Can you work these out from the model? Positions are in its coordinate system, mm. Face numbers are marked on the shaded views. A direction names the side the tool comes from. Round coordinates to 2 decimals unless told otherwise and drop trailing zeros. Loops run counter-clockwise (first coordinate to the right, second up) from the corner with the lowest first, then second, coordinate; pieces in that order, holes last. Notation, with made-up numbers: (69, 87) -> (87, 87) arc R26 cw to (87, 108) -> close; hole circle Ø9 at (62, -31). An arc over 180 degrees is marked (long way). Write each question's results on one line, items separated by ' | '.
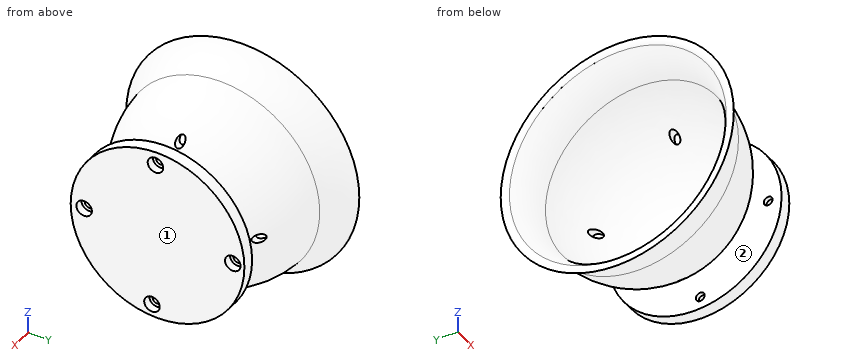
Autodesk Inventor part; units mm, degrees
ref_plane "YZ Plane" through (0, 0, 0) normal (1, 0, 0) x (0, 1, 0)
ref_plane "XZ Plane" through (0, 0, 0) normal (0, 1, 0) x (-1, 0, 0)
ref_plane "XY Plane" through (0, 0, 0) normal (0, 0, 1) x (1, 0, 0)
sketch "Sketch1" plane through (0, 0, 0) normal (0, 1, 0) x (-1, 0, 0)
  arc A0 (-48.26, 0) -> (-2.8901, -48.1734) centre (0, 0) ccw
  line L0 (0, 0) -> (2.3486, 0) construction
  arc A1 (-48.26, -15.8623) -> (-2.7486, -50.7256) centre (0, 0) ccw
  arc A2 (15.4672, -59.6495) -> (-2.7486, -50.7256) centre (-4.1531, -76.6458) ccw
  arc A3 (14.9178, -55.5155) -> (-2.8901, -48.1734) centre (-4.6642, -77.7436) ccw
  arc A4 (15.4672, -59.6495) -> (14.9178, -55.5155) centre (12.8191, -57.8979) ccw
  line L1 (31.2133, 0) -> (-72.6552, 0)
  line L2 (-48.26, 0) -> (-54.61, 0)
  line L3 (-54.61, 0) -> (-54.61, -44.45)
  line L4 (-54.61, -44.45) -> (-48.26, -44.45)
  line L5 (-48.26, -44.45) -> (-48.26, -15.8623)
  point P0 (-50.8, 0)
  dimension "d0" = 48.26
  dimension "d2" = 2.54
  dimension "d3" = 3.175
  dimension "d13" = 6.35
  dimension "d14" = 44.45
  dimension "d15" = 25.9583
  dimension "d16" = 29.6234
  dimension "d17" = 59.6495
  dimension "d18" = 55.5155
  dimension "d19" = 57.8979
  dimension "d20" = 50.6086
  dimension "d21" = 2.54
revolve "Revolution1" add sketch "Sketch1" angle 360 about axis through (-10, 0, 0) along (1, 0, 0)
hole "Hole1" at (54.61, -2.8557, -38.0756) direction (-1, 0, 0) diameter 4.4958 end through all counterbore diameter 7.9502 counterbore depth 4.1656
hole "Hole2" at (54.61, -1.0655, 37.4744) direction (-1, 0, 0) diameter 4.4958 end through all counterbore diameter 7.9502 counterbore depth 4.1656
hole "Hole3" at (54.61, -37.5872, 0.0574) direction (-1, 0, 0) diameter 4.4958 end through all counterbore diameter 7.9502 counterbore depth 4.1656
hole "Hole4" at (54.61, 38.4998, -0.1216) direction (-1, 0, 0) diameter 4.4958 end through all counterbore diameter 7.9502 counterbore depth 4.1656
properties part number "Launcher Cup"
1. If we section it at A-A (x = -0.5): List the corners of the cut face in (y, z) for me, then the cut area to 3 significant figures.
Final values:
outline: circle Ø102.22 at (0, 0); hole circle Ø97.15 at (0, 0) | area: 794 mm2
2. Please list where these lines run through material, in increasing order: line 1 (Y direction, x = -0.5, z = 4); line 2 (Z direction, x = 37, y = 14.5); line 3 (X direction, y = -20.5, z = -21.5). Write a range as from..to.
Final values:
line 1: -50.95..-48.41, 48.41..50.95 | line 2: -31.64..-27.38, 27.38..31.64 | line 3: 38.03..41.21, 48.26..54.61
3. Will these pins go through, and if not, where does the flat tip stop? pin 1 (6.5 mm diameter, centred on y = -1.07, z = 37.47, fed in from +X); pin 2 (1 mm diameter, centred on x = 15, z = 38.5, fed in from -Y); pin 3 (3.5 mm diameter, centred on y = 38.5, z = -0.12, fed in from +X); pin 4 (4 mm diameter, centred on x = -7, y = 28.5, fed in from -Z).
Final values:
pin 1: x = 50.44 | pin 2: y = -30.24 | pin 3: through | pin 4: z = -46.64
4. On a 3-axis mill with a long thin cutter (end or side, diameter ignored), from which of +Z, -Z, +X, -X, +Y, -Y can I reach the whole of each face in a straight line? I mean the marked faces 1 and 2. Say none if no direction works.
Final values:
face 1: +Z, -Z, +X, +Y, -Y | face 2: none
